```python
from build123d import *

# Parameters (mm, degrees)
SKICA1_W              = 5
SKICA1_H              = 2
ROTOVAT1_ANGLE        = 180
M3_Z_VIT1_D           = 2.5
M3_Z_VIT1_CSINK_D     = 3.05
M3_Z_VIT1_CSINK_ANGLE = 90


with BuildPart() as part:
    # Skica1 → Rotovat1 (revolve)
    with BuildSketch(Plane.XY):
        with Locations((-355.55, 23)):
            Rectangle(SKICA1_W, SKICA1_H)
    revolve(axis=Axis((-344.904513271, 0, 0), (-1, 0, 0)), revolution_arc=ROTOVAT1_ANGLE)

    # M3 závit1 (through all)
    with Locations(Plane(origin=(-355.55, 0, -24), x_dir=(-1, 0, 0), z_dir=(0, 0, -1))):
        with Locations((0, 0)):
            CounterSinkHole(M3_Z_VIT1_D / 2, M3_Z_VIT1_CSINK_D / 2, counter_sink_angle=M3_Z_VIT1_CSINK_ANGLE)


solid = part.part
```
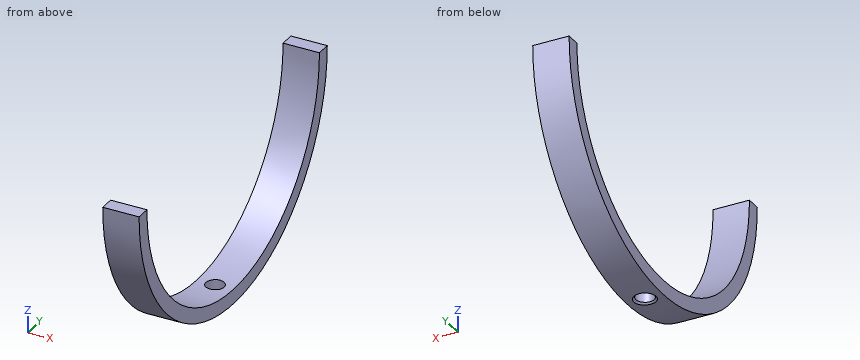
Check sheet for the modelled part. Datum: model origin and axes. Units: mm. Round coordinates to 2 decimals unless told otherwise and drop trailing zeros. Loops run counter-clockwise (first coordinate to the right, second up) from the corner with the lowest first, then second, coordinate; pieces in that order, holes last. Notation, with made-up numbers: (-24.5, 35) - (1.5, 35) arc R20 ccw to (1.5, 43) - close; hole circle Ø6 at (-13.5, 4.25). An arc over 180 degrees is marked (long way). Answer as a JSON object with one key per item and string values. Group by question number.
Q1. Sectioned sample at B-B, the plane z = -6.25. Enter the section's corners in (x, y).
Q2. Sectioned sample at C-C, the plane x = -355.55. Enter the section's corners in (y, z) (3 decimals), plus the area to 3 significant figures.
Q3. Scan lines: line 1 along X through (y, z) = (0, -22.95); line 2 along Y through (x, z) = (-356.15, -10.5); line 3 along Y through (x, z) = (-354.5, -8). Record each from-to range of solid material in increasing order. Write a range as [from, to].
Q4. Sectioned sample at D-D, the plane z = -2.5. Enter the section's corners in (x, y).
Q5. Gauge pin test, flat ends, axial feed: P1, Ø1.5, axis at x = -354.5, y = 6.5, coming from the +Z side; P2, Ø2, axis at x = -355.5, z = -12, coming from the -Y side; P3, Ø2, axis at x = -356.5, z = -2.5, coming from the +Y side. Record the tip position at first contact, or that the pin passes through.
Q6. Sectioned sample at A-A, the plane y = 0. Enter the section's corners in (x, z) (3 decimals).
Solution:
{
 "1": {"outline": "(-358.05, -23.17) - (-353.05, -23.17) - (-353.05, -21.09) - (-358.05, -21.09) - close; (-358.05, 21.09) - (-353.05, 21.09) - (-353.05, 23.17) - (-358.05, 23.17) - close"},
 "2": {"outline": "(-24, 0) arc R24 ccw to (-1.479, -23.954) - (-1.25, -23.725) - (-1.25, -21.964) arc R22 cw to (-22, 0) - close; (1.25, -23.725) - (1.479, -23.954) arc R24 ccw to (24, 0) - (22, 0) arc R22 cw to (1.25, -21.964) - close", "area": "139 mm²"},
 "3": {"line 1": "x = [-358.05, -356.8], [-354.3, -353.05]", "line 2": "y = [-21.58, -19.33], [19.33, 21.58]", "line 3": "y = [-22.63, -20.49], [20.49, 22.63]"},
 "4": {"outline": "(-358.05, -23.87) - (-353.05, -23.87) - (-353.05, -21.86) - (-358.05, -21.86) - close; (-358.05, 21.86) - (-353.05, 21.86) - (-353.05, 23.87) - (-358.05, 23.87) - close"},
 "5": {"P1": "stops at z = -20.77", "P2": "stops at y = -21.33", "P3": "stops at y = 23.95"},
 "6": {"outline": "(-358.05, -24) - (-357.075, -24) - (-356.8, -23.725) - (-356.8, -22) - (-358.05, -22) - close; (-354.3, -23.725) - (-354.025, -24) - (-353.05, -24) - (-353.05, -22) - (-354.3, -22) - close"}
}
